Input: part model. Units: mm. Frame: model coordinates. A direction names the side the tool comes from. Round coordinates to 2 decimals unless told otherwise and drop trailing zeros. Write each loop counter-clockwise with the first axis right and the second up, starting at its lowest first coordinate (ties: lowest second). Pieces come first, ordered by that corner, then holes. Notation, with made-up numbers: M -26.75,56.5 L 11.25,56.5 A22 cw 11.25,91.5 Z; hole C -12,-38 d2. An arc over 180 degrees is marked long. Use one line per item in the form item = value. Start each with the question number.
Autodesk Inventor part; units mm, degrees
ref_plane "YZ Plane" through (0, 0, 0) normal (1, 0, 0) x (0, 1, 0)
ref_plane "XZ Plane" through (0, 0, 0) normal (0, 1, 0) x (-1, 0, 0)
ref_plane "XY Plane" through (0, 0, 0) normal (0, 0, 1) x (1, 0, 0)
sketch "Sketch1" plane through (0, 0, 0) normal (0, 0, 1) x (1, 0, 0)
  circle A0 centre (0, 0) radius 3.125
  circle A1 centre (0, 0) radius 4.025
  circle A2 centre (0, 0) radius 7.5
  dimension "d0" = 6.25
  dimension "d1" = 0.9
  dimension "d2" = 15
extrude "Extrusion1" add sketch "Sketch1" along normal blind 2 contours A1 | A2
extrude "Extrusion2" add sketch "Sketch1" against normal blind 16 contours A1
sketch "Sketch2" plane through (0, 0, -16) normal (0, 0, -1) x (-1, 0, 0)
  circle A0 centre (0, 0) radius 4.025
  circle A1 centre (0, 0) radius 7.5
  circle A2 centre (0, 0) radius 3.125
  circle A3 centre (0, 0) radius 1.5
  dimension "d9" = 3
extrude "Extrusion3" add sketch "Sketch2" along normal blind 4 contours A0 | A1 | A2
sketch "Sketch3" plane through (0, 0, -20) normal (0, 0, -1) x (-1, 0, 0)
  circle A0 centre (0, 0) radius 1.5
  circle A1 centre (0, 0) radius 7.5
  circle A2 centre (0, 11) radius 1.5
  circle A3 centre (0, 11) radius 4
  circle A4 centre (0, 0) radius 7.5
  line L0 (4, 11) -> (7.0537, 2.5487)
  line L1 (-4, 11) -> (-7.0537, 2.5487)
  dimension "d10" = 3
  dimension "d11" = 11
  dimension "d12" = 8
  dimension "d41" = 0
extrude "Extrusion4" add sketch "Sketch3" against normal blind 3
pattern_circular "Circular Pattern1" count 2 over 360 about axis through (0, 0, -16) along (0, 0, -1) of "Extrusion4"
extrude "Extrusion5" add sketch "Sketch2" against normal blind 2 contours A1
fillet "Fillet1" radius 10 4 edges at (-4, 11, -18.5) (4, 11, -18.5) (-4, -11, -18.5) (4, -11, -18.5)
chamfer "Chamfer1" distance 1 angle 45 2 edges at (-4.025, 0, -14) (-4.025, 0, 0)
sketch "Sketch4" plane through (0, 0, 2) normal (0, 0, 1) x (1, 0, 0)
  circle A0 centre (0, 0) radius 3.125
  circle A1 centre (0, 0) radius 7.5
  circle A2 centre (0, 0) radius 7.5
  line L0 (2.75, 6.9776) -> (2.75, 15)
  line L1 (2.75, 15) -> (-2.75, 15)
  line L2 (-2.75, 15) -> (-2.75, 6.9776)
  circle A3 centre (0, 4.8) radius 0.5
  circle A4 centre (0, 7.4) radius 0.5
  circle A5 centre (0, 10) radius 0.5
  circle A6 centre (0, 12.6) radius 0.5
  circle A7 centre (0, 0) radius 4.025
  dimension "d24" = 2.75
  dimension "d25" = 2.75
  dimension "d26" = 7.5
  dimension "d27" = 1
  dimension "d28" = 4.8
  dimension "d31" = 2.6
extrude "Extrusion6" add sketch "Sketch4" against normal blind 2 contours A1 A4 L2 L1 L0 | A1 A4 picked at (0, 7.6321)
extrude "Extrusion7" cut sketch "Sketch4" against normal blind 3 contours A4 A1 | A1 A4 | A3 picked at (-0.014, 7.2994) picked at (0, 7.6321)
fillet "Fillet2" radius 2 4 edges at (2.75, 6.9776, 1) (-2.75, 6.9776, 1) (-2.75, 15, 1) (2.75, 15, 1)
properties part number "3DP_ABS_Solenoid_Actuator_Body" material "ABS Plastic"
Item 1: Cut plane B-B (z = -3.5). Output: boundary loops of the cut face in (x, y) (3 decimals).
Item 2: Cut plane C-C (x = -6). Output: boundary loops of the cut face in (y, z), plus the area to 3 significant figures.
Item 3: Cut plane A-A (y = 0). Output: boundary loops of the cut face in (x, z) (3 decimals), plus the area to 3 significant figures.
Item 4: Reachability of faces 5 (the face through (0, 9, -17)), 6 (the face through (3.03, 7.21, 0.99)), 7 (the face through (0, 15, -19)), 8 (the face through (-2.18, 14.4, 0.99)) from +Z, -Z, +X, -X, +Y, -Y: full face, straight path, thin tool, end or side. Return the list, or none.
Item 5: First-contact query: pin 1 (4 mm diameter, centred on x = 0, y = 0, fed in from -Z); pin 2 (1.9 mm diameter, centred on x = -1, y = -1, fed in from +Z); pin 3 (1 mm diameter, centred on x = 1.5, z = -11.5, fed in from +Y); pin 4 (1.6 mm diameter, centred on y = 10, z = 1, fed in from +X). Flat tips, straight axial feed; report the tip coordinate or a pass-through.
Item 6: Draft query along Z for faces 1 (the face through (0, -9, -17)), 2 (the face through (0.231, 12.156, 1.014)), 3 (the face through (0, 6, 0)), 4 (the face through (-2, 0, -20)). Return one class per face: +Z half, -Z half, draft (parallel to the pull), parting line (faces both ways), or undercut.
Item 7: Cut plane D-D (y = -10.5). Output: boundary loops of the cut face in (x, z), plus the area to 3 significant figures.
Item 8: Ray query, line 1 (Y direction, x = 0, z = 0.9) (3 decimals); line 2 (Y direction, x = 0, z = -4) (3 decimals); line 3 (Y direction, x = 0.5, z = -19). Return the intervals inside material, ascending. Write a range as from..to.
Final values:
q1.outline = C 0,0 d8.05; hole C 0,0 d6.25
q2.outline = M -5.46,-20 L 5.46,-20 L 5.46,-17 L 4.5,-17 L 4.5,-14 L -4.5,-14 L -4.5,-17 L -5.46,-17 Z; M -4.5,0 L 4.5,0 L 4.5,2 L -4.5,2 Z
q2.area = 77.8 mm^2
q3.outline = M -7.5,-20 L -1.5,-20 L -1.5,-16 L -3.125,-16 L -3.125,2 L -7.5,2 L -7.5,0 L -5.025,0 L -4.025,-1 L -4.025,-13 L -5.025,-14 L -7.5,-14 Z; M 1.5,-20 L 7.5,-20 L 7.5,-14 L 5.025,-14 L 4.025,-13 L 4.025,-1 L 5.025,0 L 7.5,0 L 7.5,2 L 3.125,2 L 3.125,-16 L 1.5,-16 Z
q3.area = 110 mm^2
q4.face_5 = +Y
q4.face_6 = +Z, +X, +Y
q4.face_7 = -Z, +Y
q4.face_8 = +Z, -X, +Y
q5.pin_1 = -20
q5.pin_2 = -16
q5.pin_3 = 3.9
q5.pin_4 = 2.75
q6.face_1 = +Z half
q6.face_2 = draft
q6.face_3 = undercut
q6.face_4 = -Z half
q7.outline = M -4.2,-20 L -1.41,-20 L -1.41,-17 L -4.2,-17 Z; M 1.41,-20 L 4.2,-20 L 4.2,-17 L 1.41,-17 Z
q7.area = 16.7 mm^2
q8.line_1 = -7.5..-3.125, 3.125..4.3, 5.3..6.9, 7.9..9.5, 10.5..12.1, 13.1..15
q8.line_2 = -4.025..-3.125, 3.125..4.025
q8.line_3 = -14.97..-12.41, -9.59..-1.41, 1.41..9.59, 12.41..14.97
